For this review, use the dimensioned drawing (mm, ordinates from the lowest corner) and the shaded views. A direction names the side the tool comes from. Give positions to 0.01 mm unless a question says otherwise; leave off trailing zeros. Loops run counter-clockwise (first coordinate to the right, second up) from the corner with the lowest first, then second, coordinate; pieces in that order, holes last. Notation, with made-up numbers: (18, 75) -> (62, 75) arc R14 ccw to (62, 100) -> close; hole circle Ø8 at (71.25, 3). An arc over 180 degrees is marked (long way). Use a Markdown table: item, result. Add a question column.
1. Draft analysis for pull direction Z (two halves, no side actions). For the marked faces 1, 2 and 3, state which applies: pulls with the +Z half, pulls with the -Z half, needs draft (parallel to the pull), parting line crosses it, or undercut.
2. To check wall thickness, follow line 1 (Y direction, x = 85, z = 74.5) (1 decimal); line 2 (Y direction, x = 85, z = 75) (1 decimal); line 3 (Y direction, x = 85, z = 64) (1 decimal). State the ranges of each line that lie inside material, in increasing order.
3. Add section D-D (z = 35). State the section outline as (x, y) points (3 decimals).
4. For the marked faces 4, 5, 6 and 7, list the 3-axis set-ups (+Z, -Z, +X, -X, +Y, -Y) from which the entire face can be reached by the end or side of a thin tool; tool diameter is ignored.
5. Add section C-C (z = 68). State the section outline as (x, y) points (3 decimals).
6. For pin 1 Ø2 at (x, z) = (70, 24) entering from +Y; pin 2 Ø9 at (x, y) = (87, 46.5) entering from +Z; pin 3 Ø6 at (x, z) = (125, 83.5) entering from -Y (3 decimals), all flat-tipped, find the tip position at first contact; note any pin that passes through.
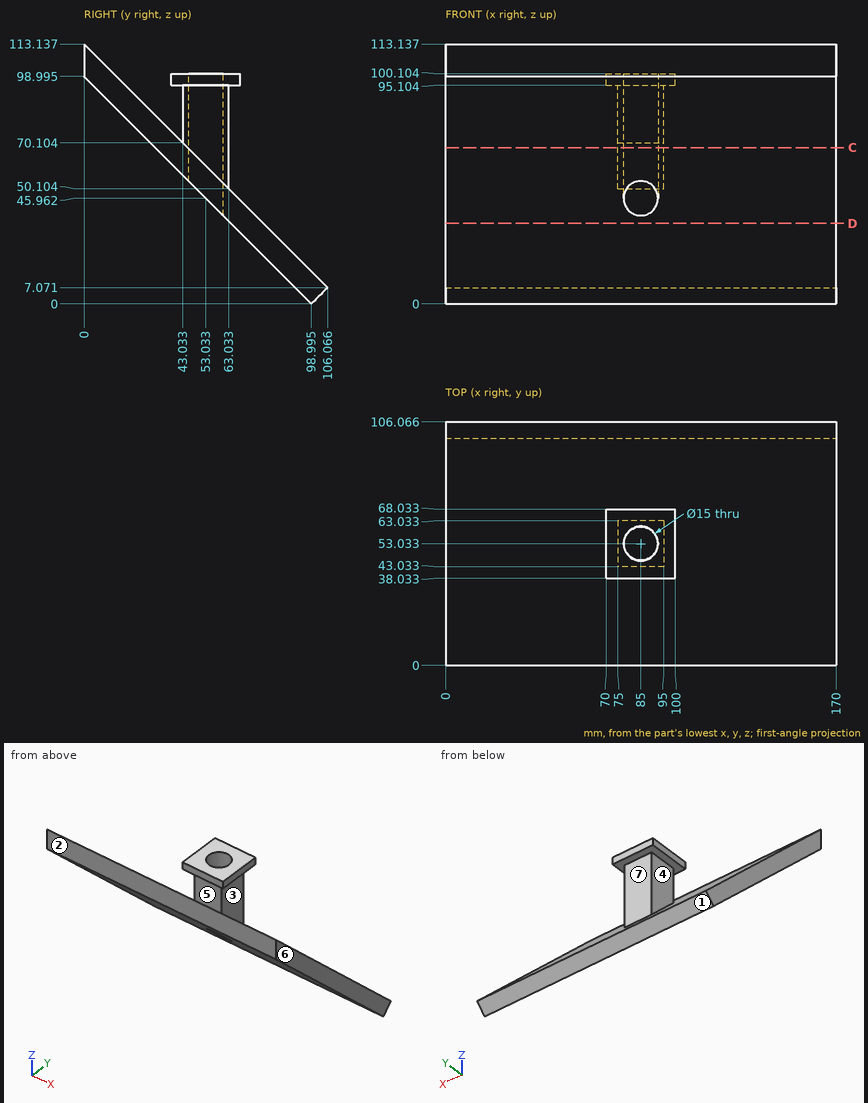
Taken from the geometry:
| question | item | result |
|---|---|---|
| 1 | face 1 | pulls with the -Z half |
| 1 | face 2 | needs draft |
| 1 | face 3 | undercut |
| 2 | line 1 | y = 24.5 to 38.6, 43 to 45.5, 60.5 to 63 |
| 2 | line 2 | y = 24 to 38.1, 43 to 45.5, 60.5 to 63 |
| 2 | line 3 | y = 35 to 45.5, 60.5 to 63 |
| 3 | outline | (0, 63.995) -> (170, 63.995) -> (170, 78.137) -> (0, 78.137) -> close |
| 4 | face 4 | -X, +Y |
| 4 | face 5 | +X, -X |
| 4 | face 6 | +Z, -Z, +X, +Y, -Y |
| 4 | face 7 | +X, -X, +Y |
| 5 | outline | (0, 30.995) -> (170, 30.995) -> (170, 45.137) -> (95, 45.137) -> (95, 63.033) -> (75, 63.033) -> (75, 45.137) -> (0, 45.137) -> close; hole circle Ø15 at (85, 53.033) |
| 6 | pin 1 | stops at y = 90.14 |
| 6 | pin 2 | stops at z = 100.1 |
| 6 | pin 3 | stops at y = 12.495 |
